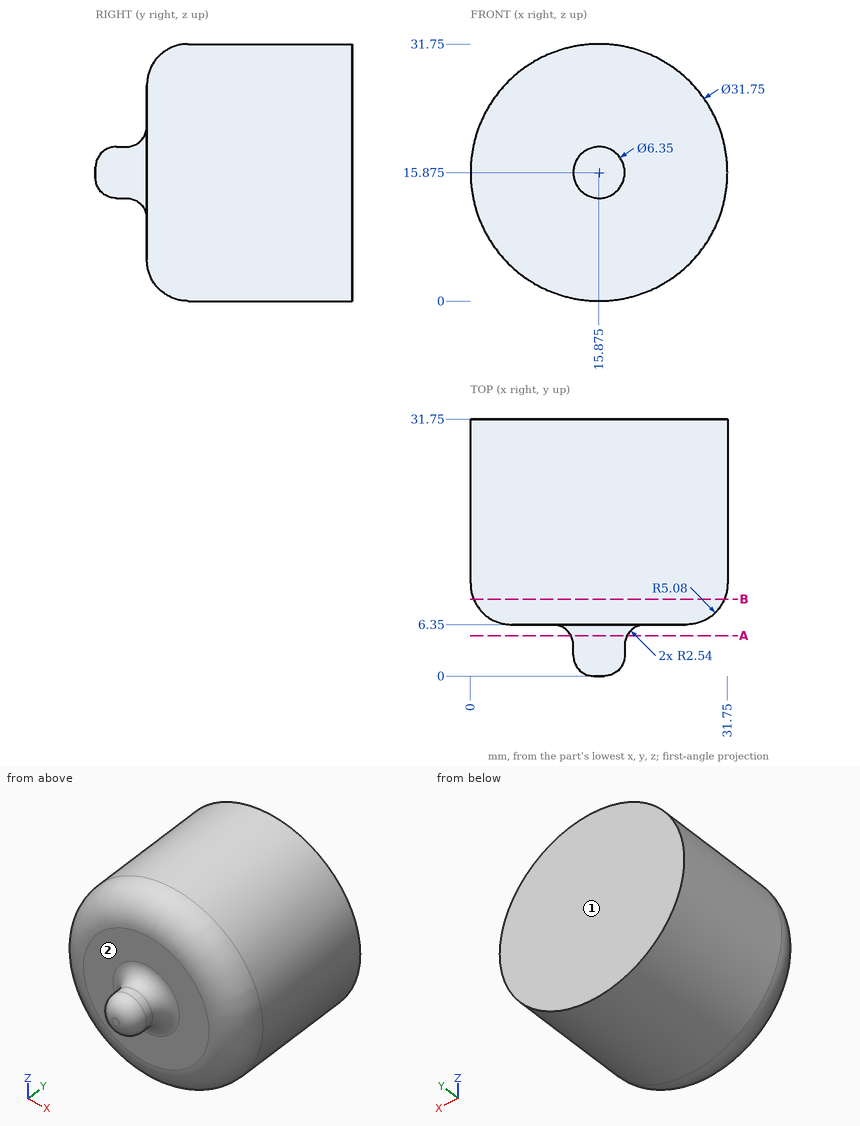
Design review of the part shown in the three views and the two pictorial views. Dimensions are in mm from the part's minimum x, y and z. A direction names the side the tool comes from. Round coordinates to 2 decimals unless told otherwise and drop trailing zeros. Loops run counter-clockwise (first coordinate to the right, second up) from the corner with the lowest first, then second, coordinate; pieces in that order, holes last. Notation, with made-up numbers: M -3.75,53.5 L 41.25,53.5 A3 ccw 41.25,57.5 Z; hole C 79,-4 d11. An arc over 180 degrees is marked long. Put each result on its own line as item: value.
Q1. Consider section A-A, the plane y = 5. Give the boundary of the cut face in (x, z) (3 decimals), then the cut area to 3 significant figures.
Result set:
outline: C 15.875,15.875 d6.942
area: 37.8 mm²
Q2. Machinability: for the marked faces 1 and 2, which of the approach directions +Z, -Z, +X, -X, +Y, -Y give a long, thin tool a straight path to every point of the face, cutting with its end or side? Answer none if there is none.
Result set:
face 1: +Z, -Z, +X, -X, +Y
face 2: -Y
Q3. For pin 1 (3 mm diameter, centred on y = 17, z = 27.5, fed in from +X); pin 2 (2 mm diameter, centred on x = 19.5, y = 24, fed in from -Z); pin 3 (6 mm diameter, centred on y = 7.5, z = 20, fed in from -X); pin 4 (1.5 mm diameter, centred on x = 16.5, z = 16.5, fed in from -Y), all flat-tipped, find the tip position at first contact; note any pin that passes through.
Result set:
pin 1: stops at x = 28.1
pin 2: stops at z = 0.22
pin 3: stops at x = 0.4
pin 4: stops at y = 0
Q4. Consider section B-B, the plane y = 9.5. Give the boundary of the cut face in (x, z) (3 decimals).
Result set:
outline: C 15.875,15.875 d30.988
Q5. To check wall thickness, follow L1, parallel to Y at x = 5.5, z = 13.5; L2, parallel to Y at x = 7, z = 7.5; L3, parallel to Z at x = 3.5, y = 13. State the ranges of each line that lie inside material, in increasing order.
Result set:
L1: y = 6.35 to 31.75
L2: y = 6.55 to 31.75
L3: z = 5.93 to 25.82
